```python
from build123d import *

# Parameters (mm, degrees)
BOSS_EXTRUDE1_DEPTH = 20
SKETCH1_7_R         = 20
BOSS_EXTRUDE5_DEPTH = 5
SKETCH4_R           = 15
SKETCH4_R_2         = 14.5
BOSS_EXTRUDE6_DEPTH = 10
SKETCH5_R           = 3
CUT_EXTRUDE1_DEPTH  = 20


with BuildPart() as part:
    # Sketch1 → Boss-Extrude1 (new body)
    with BuildSketch(Plane.XY):
        with BuildLine():
            ThreePointArc((-4.708142303, 13.714350005), (-6.901237199, 12.752369392), (-8.906084334, 11.442537386))
            Line((-8.906084334, 11.442537386), (-9.21319069, 11.837107641))
            ThreePointArc((-9.21319069, 11.837107641), (-11.03585866, 10.159223574), (-12.557497174, 8.204222372))
            Line((-12.557497174, 8.204222372), (-12.138913935, 7.930748293))
            ThreePointArc((-12.138913935, 7.930748293), (-13.278713236, 5.824583657), (-14.056303856, 3.559539564))
            Line((-14.056303856, 3.559539564), (-14.541003989, 3.682282307))
            ThreePointArc((-14.541003989, 3.682282307), (-14.948767395, 1.238690182), (-14.948767395, -1.238690182))
            Line((-14.948767395, -1.238690182), (-14.450475149, -1.197400509))
            ThreePointArc((-14.450475149, -1.197400509), (-14.056303856, -3.559539564), (-13.278713236, -5.824583657))
            Line((-13.278713236, -5.824583657), (-13.7365999, -6.02543137))
            ThreePointArc((-13.7365999, -6.02543137), (-12.557497174, -8.204222372), (-11.03585866, -10.159223574))
            Line((-11.03585866, -10.159223574), (-10.667996705, -9.820582789))
            ThreePointArc((-10.667996705, -9.820582789), (-8.906084334, -11.442537386), (-6.901237199, -12.752369392))
            Line((-6.901237199, -12.752369392), (-7.139210896, -13.192106268))
            ThreePointArc((-7.139210896, -13.192106268), (-4.870492038, -14.187258626), (-2.468918854, -14.795419551))
            Line((-2.468918854, -14.795419551), (-2.386621559, -14.302238899))
            ThreePointArc((-2.386621559, -14.302238899), (0, -14.5), (2.386621559, -14.302238899))
            Line((2.386621559, -14.302238899), (2.468918854, -14.795419551))
            ThreePointArc((2.468918854, -14.795419551), (4.870492038, -14.187258626), (7.139210896, -13.192106268))
            Line((7.139210896, -13.192106268), (6.901237199, -12.752369392))
            ThreePointArc((6.901237199, -12.752369392), (8.906084334, -11.442537386), (10.667996705, -9.820582789))
            Line((10.667996705, -9.820582789), (11.03585866, -10.159223574))
            ThreePointArc((11.03585866, -10.159223574), (12.557497174, -8.204222372), (13.7365999, -6.02543137))
            Line((13.7365999, -6.02543137), (13.278713236, -5.824583657))
            ThreePointArc((13.278713236, -5.824583657), (14.056303856, -3.559539564), (14.450475149, -1.197400509))
            Line((14.450475149, -1.197400509), (14.948767395, -1.238690182))
            ThreePointArc((14.948767395, -1.238690182), (14.948767395, 1.238690182), (14.541003989, 3.682282307))
            Line((14.541003989, 3.682282307), (14.056303856, 3.559539564))
            ThreePointArc((14.056303856, 3.559539564), (13.278713236, 5.824583657), (12.138913935, 7.930748293))
            Line((12.138913935, 7.930748293), (12.557497174, 8.204222372))
            ThreePointArc((12.557497174, 8.204222372), (11.03585866, 10.159223574), (9.21319069, 11.837107641))
            Line((9.21319069, 11.837107641), (8.906084334, 11.442537386))
            ThreePointArc((8.906084334, 11.442537386), (6.901237199, 12.752369392), (4.708142303, 13.714350005))
            Line((4.708142303, 13.714350005), (4.870492038, 14.187258626))
            ThreePointArc((4.870492038, 14.187258626), (0, 15), (-4.870492038, 14.187258626))
            Line((-4.870492038, 14.187258626), (-4.708142303, 13.714350005))
        make_face()
    extrude(amount=BOSS_EXTRUDE1_DEPTH)

    # Sketch1_7 → Boss-Extrude5 (add)
    with BuildSketch(Plane.XY):
        Circle(SKETCH1_7_R)
    extrude(amount=-BOSS_EXTRUDE5_DEPTH)

    # Sketch4 → Boss-Extrude6 (add)
    with BuildSketch(Plane.XY):
        with Locations(Location((0, 0, 0), (0, 0, 184.736842105))):
            Circle(SKETCH4_R)
        Circle(SKETCH4_R_2, mode=Mode.SUBTRACT)
    extrude(amount=BOSS_EXTRUDE6_DEPTH)

    # Sketch5 → Cut-Extrude1 (cut)
    with BuildSketch(Plane.XY.offset(20)):
        Circle(SKETCH5_R)
    extrude(amount=-CUT_EXTRUDE1_DEPTH, mode=Mode.SUBTRACT)


solid = part.part
```
The listing builds one solid part. Answer for the finished solid, in the listing's coordinates (mm). A direction names the side the tool comes from. Give positions to 0.01 mm unless a question says otherwise; leave off trailing zeros. Loops run counter-clockwise (first coordinate to the right, second up) from the corner with the lowest first, then second, coordinate; pieces in that order, holes last. Notation, with made-up numbers: (-1.5, -39.5) - (51.5, -39.5) arc R28 ccw to (51.5, -0.5) - close; hole circle Ø5 at (26, 80). An arc over 180 degrees is marked (long way). Return JSON: item names as keys, results as strings. Group by question number.
1. Find section B-B (x = 0). Write down the section's boundary in (y, z), then the cut area to 3 significant figures.
2. Find section D-D (z = -2.25). Write down the section's boundary in (x, y).
3. Find section A-A (z = 5.5). Write down the section's boundary in (x, y).
4. Find section C-C (y = 0). Write down the section's boundary in (x, z), then the cut area to 3 significant figures.
5. Given pin 1 Ø2 at (x, z) = (-3.5, 10.5) entering from +Y; pin 2 Ø1 at (x, z) = (11.5, 7.5) entering from -Y; pin 3 Ø1.8 at (x, y) = (-1, 1) entering from +Z, each flat-ended and moving along its own axis, determine where each tip first touches the part or whether it passes through.
6. Determine the mould class of faces 3 (the flat face through (3, 15, 0)), 4 (the cylindrical face through (-4.336, -19.524, -2.465)), 5 (the cylindrical face through (0, -14.5, 14.9)) for opening direction X: pulls with the +X half, pulls with the -X half, needs draft (parallel to the pull), parting line crosses it, or undercut.
7. Straight lines are drawn through the part: line 1 (Y direction, x = 0, z = 10.5); line 2 (Y direction, x = 0, z = 7.5); line 3 (Z direction, x = 10, y = -11). For each, find the intervals that lie inside material, in ascending order. Write a range as [from, to].
8. Which of the six approach directions +Z, -Z, +X, -X, +Y, -Y give full straight-line access (tool end or side, diameter ignored) to faces 1 (the cylindrical face through (-3, 0, 10)), 2 (the flat face through (-4, 0, 20))?
Verdict:
{
 "1": {"outline": "(-20, -5) - (20, -5) - (20, 0) - (15, 0) - (15, 20) - (3, 20) - (3, 0) - (-3, 0) - (-3, 20) - (-14.5, 20) - (-14.5, 10) - (-15, 10) - (-15, 0) - (-20, 0) - close", "area": "675 mm^2"},
 "2": {"outline": "circle Ø40 at (0, 0)"},
 "3": {"outline": "circle Ø30 at (0, 0); hole circle Ø6 at (0, 0)"},
 "4": {"outline": "(-20, -5) - (20, -5) - (20, 0) - (15, 0) - (15, 20) - (3, 20) - (3, 0) - (-3, 0) - (-3, 20) - (-15, 20) - (-15, 0) - (-20, 0) - close", "area": "680 mm^2"},
 "5": {"pin 1": "stops at y = 14.79", "pin 2": "stops at y = -10.2", "pin 3": "stops at z = 0"},
 "6": {"face 3": "needs draft", "face 4": "parting line crosses it", "face 5": "undercut"},
 "7": {"line 1": "y = [-14.5, -3], [3, 15]", "line 2": "y = [-15, -3], [3, 15]", "line 3": "z = [-5, 10]"},
 "8": {"face 1": "+Z", "face 2": "+Z, +X, -X, +Y, -Y"}
}
